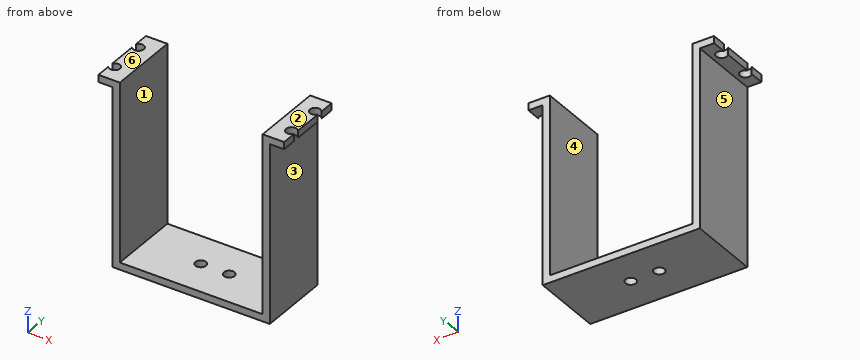
from build123d import *

# Parameters (mm, degrees)
ESQUISSE1_W             = 44
ESQUISSE1_H             = 20
BOSS_EXTRU_1_DEPTH      = 2
ESQUISSE2_W             = 2
ESQUISSE2_H             = 20
BOSS_EXTRU_2_DEPTH      = 50
ESQUISSE3_W             = 2
ESQUISSE3_H             = 20
BOSS_EXTRU_3_DEPTH      = 4
ESQUISSE4_W             = 2
ESQUISSE4_H             = 20
BOSS_EXTRU_4_DEPTH      = 4
ESQUISSE5_R             = 1.5
ENL_V_MAT_EXTRU_1_DEPTH = 4
ESQUISSE6_R             = 1.5
ENL_V_MAT_EXTRU_2_DEPTH = 4


with BuildPart() as part:
    # Esquisse1 → Boss.-Extru.1 (new body)
    with BuildSketch(Plane.XY):
        with Locations((22, 10)):
            Rectangle(ESQUISSE1_W, ESQUISSE1_H)
    extrude(amount=BOSS_EXTRU_1_DEPTH)

    # Esquisse2 → Boss.-Extru.2 (add)
    with BuildSketch(Plane.XY.offset(2)):
        with Locations((1, 10)):
            Rectangle(ESQUISSE2_W, ESQUISSE2_H)
        with Locations((43, 10)):
            Rectangle(ESQUISSE2_W, ESQUISSE2_H)
    extrude(amount=BOSS_EXTRU_2_DEPTH)

    # Esquisse3 → Boss.-Extru.3 (add)
    with BuildSketch(Plane.ZY):
        with Locations((51, 10)):
            Rectangle(ESQUISSE3_W, ESQUISSE3_H)
    extrude(amount=BOSS_EXTRU_3_DEPTH)

    # Esquisse4 → Boss.-Extru.4 (add)
    with BuildSketch(Plane(origin=(44, 0, 0), x_dir=(0, 0, -1), z_dir=(1, 0, 0))):
        with Locations((-51, 10)):
            Rectangle(ESQUISSE4_W, ESQUISSE4_H)
    extrude(amount=BOSS_EXTRU_4_DEPTH)

    # Esquisse5 → Enlèv. mat.-Extru.1 (cut)
    with BuildSketch(Plane.XY.offset(2)):
        with Locations((18, 10)):
            Circle(ESQUISSE5_R)
        with Locations((26, 10)):
            Circle(ESQUISSE5_R)
    extrude(amount=-ENL_V_MAT_EXTRU_1_DEPTH, mode=Mode.SUBTRACT)

    # Esquisse6 → Enlèv. mat.-Extru.2 (cut)
    with BuildSketch(Plane.XY.offset(52)):
        with Locations((46.75, 15)):
            Circle(ESQUISSE6_R)
        with Locations((46.75, 5)):
            Circle(ESQUISSE6_R)
        with Locations((-2.75, 15)):
            Circle(ESQUISSE6_R)
        with Locations((-2.75, 5)):
            Circle(ESQUISSE6_R)
    extrude(amount=-ENL_V_MAT_EXTRU_2_DEPTH, mode=Mode.SUBTRACT)


solid = part.part
Check sheet for the modelled part. Datum: model origin and axes. Units: mm. Face numbers are marked on the shaded views. A direction names the side the tool comes from. Give positions to 0.01 mm unless a question says otherwise; leave off trailing zeros. Write each loop counter-clockwise with the first axis right and the second up, starting at its lowest first coordinate (ties: lowest second). Pieces come first, ordered by that corner, then holes. Notation, with made-up numbers: (33, 46.25) -> (47, 46.25) arc R19 cw to (47, 74.25) -> close; hole circle Ø2 at (38.5, 87). An arc over 180 degrees is marked (long way). One line per item, written item: value. Start each with the question number.
Item 1: Section check B-B on z = 48. Record the cut outline in (x, y).
Item 2: Draft check along X on the marked faces 1, 2 and 3. Enter one of: +X half, -X half, draft (parallel to the pull), parting line (faces both ways), or undercut.
Item 3: Material ranges on probe 1 along Y at (x, z) = (-2.75, 51.55); probe 2 along X at (y, z) = (16.75, 48.5); probe 3 along X at (y, z) = (5, 51.25), recorded low to high. Write a range as from..to.
Item 4: Tool access check on the marked faces 4, 5 and 6. Record the directions out of +Z, -Z, +X, -X, +Y, -Y that give a thin tool (end or side, any length) a straight path to the whole face; none if there is none.
Item 5: Section check D-D on y = 15. Record the cut outline in (x, z), then the cut area to 3 significant figures.
Item 6: Section check A-A on x = 46.75. Record the cut outline in (y, z), then the cut area to 3 significant figures.
Item 7: Gauge pin test, flat ends, axial feed: pin 1 (3 mm diameter, centred on x = 11, y = 9, fed in from +Z); pin 2 (3.5 mm diameter, centred on x = -2.75, y = 15, fed in from -Z); pin 3 (1 mm diameter, centred on y = 9.5, z = 7.5, fed in from +X). Record the tip position at first contact, or that the pin passes through.
Item 8: Section check C-C on x = 18. Record the cut outline in (y, z), then the cut area to 3 significant figures.
Results list:
1. outline: (0, 0) -> (2, 0) -> (2, 20) -> (0, 20) -> close; (42, 0) -> (44, 0) -> (44, 20) -> (42, 20) -> close
2. face 1: undercut
2. face 2: draft
2. face 3: +X half
3. probe 1: 0..3.5, 6.5..13.5, 16.5..20
3. probe 2: 0..2, 42..44
3. probe 3: -1.25..2, 42..45.25
4. face 4: +Z, +Y, -Y
4. face 5: -Z, -X, +Y, -Y
4. face 6: +Z, +X, -X, +Y, -Y
5. outline: (-1.25, 50) -> (0, 50) -> (0, 0) -> (44, 0) -> (44, 50) -> (45.25, 50) -> (45.25, 52) -> (42, 52) -> (42, 2) -> (2, 2) -> (2, 52) -> (-1.25, 52) -> close
5. area: 293 mm²
6. outline: (0, 50) -> (3.5, 50) -> (3.5, 52) -> (0, 52) -> close; (6.5, 50) -> (13.5, 50) -> (13.5, 52) -> (6.5, 52) -> close; (16.5, 50) -> (20, 50) -> (20, 52) -> (16.5, 52) -> close
6. area: 28.0 mm²
7. pin 1: z = 2
7. pin 2: z = 50
7. pin 3: x = 44
8. outline: (0, 0) -> (8.5, 0) -> (8.5, 2) -> (0, 2) -> close; (11.5, 0) -> (20, 0) -> (20, 2) -> (11.5, 2) -> close
8. area: 34.0 mm²
